Part print with two shaded views. Sizes in mm from the minimum x, y, z corner. A direction names the side the tool comes from. Round coordinates to 2 decimals unless told otherwise and drop trailing zeros. Order: outer loops, then holes, each group sorted by start corner. A loop starts at its lowest first (then second) coordinate and runs counter-clockwise, first axis right, second up. Notation, with made-up numbers: (28.5, 84.5) -> (36.5, 84.5) arc R15 cw to (36.5, 95.5) -> close; hole circle Ø2 at (50, 39.5). An arc over 180 degrees is marked (long way). Answer as a JSON object with one key per item and string values.
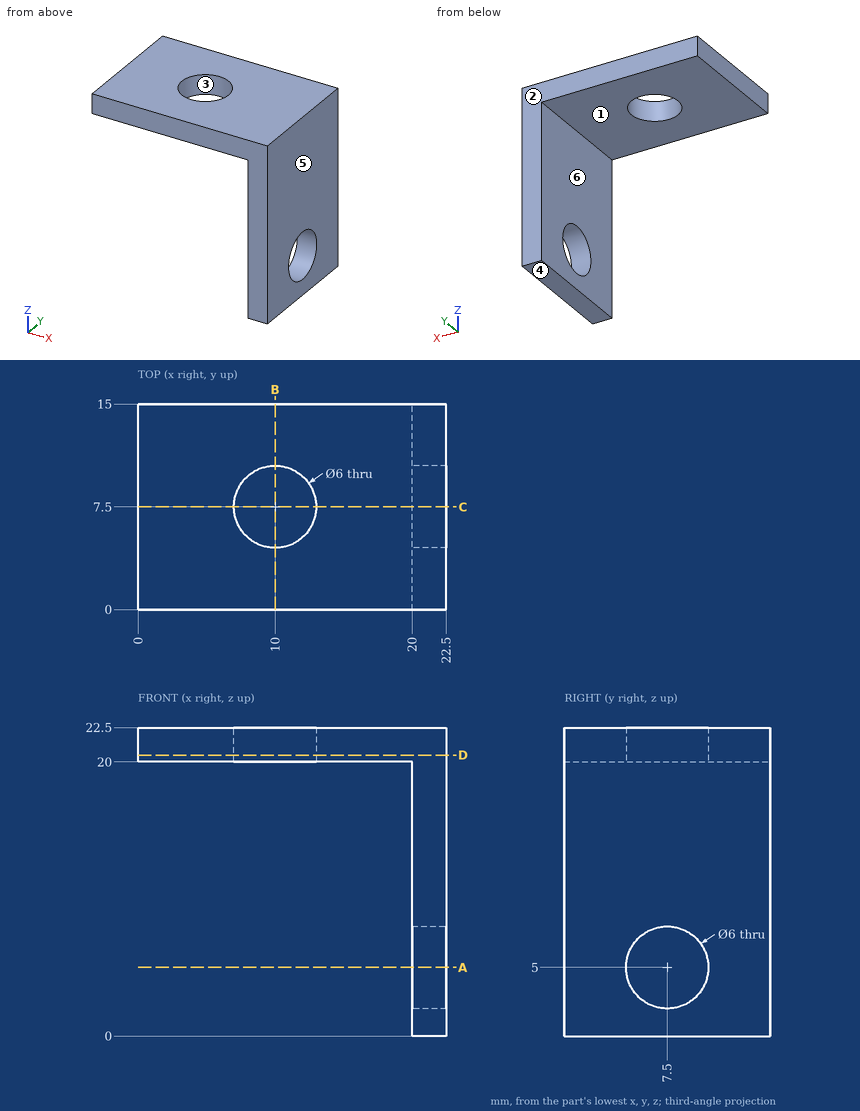
1) Cut at C-C, the plane y = 7.5. Give the cut face in (x, z).
Checked values:
{"outline": "(0, 20) -> (7, 20) -> (7, 22.5) -> (0, 22.5) -> close; (13, 20) -> (20, 20) -> (20, 8) -> (22.5, 8) -> (22.5, 22.5) -> (13, 22.5) -> close; (20, 0) -> (22.5, 0) -> (22.5, 2) -> (20, 2) -> close"}
2) Cut at D-D, the plane z = 20.5. Give the cut face in (x, y), plus the area to 3 significant figures.
Checked values:
{"outline": "(0, 0) -> (22.5, 0) -> (22.5, 15) -> (0, 15) -> close; hole circle Ø6 at (10, 7.5)", "area": "309 mm²"}
3) Probe L1, parallel to Y at x = 21.8, z = 5; L2, parallel to Z at x = 16.75, y = 3.25. List the from-to ranges inside material, lowest first. Write a range as from..to.
Checked values:
{"L1": "y = 0..4.5, 10.5..15", "L2": "z = 20..22.5"}
4) Cut at A-A, the plane z = 5. Give the cut face in (x, y), plus the area to 3 significant figures.
Checked values:
{"outline": "(20, 0) -> (22.5, 0) -> (22.5, 4.5) -> (20, 4.5) -> close; (20, 10.5) -> (22.5, 10.5) -> (22.5, 15) -> (20, 15) -> close", "area": "22.5 mm²"}
5) Which spindle directions (+Z, -Z, +X, -X, +Y, -Y) get a long thin tool onto all of the face, cutting with end or side? Do the marked faces 1 and 2. Say none if no direction does.
Checked values:
{"face 1": "-Z, -X, +Y, -Y", "face 2": "+Z, -Z, +X, -X, +Y"}
6) Cut at B-B, the plane x = 10. Give the cut face in (y, z).
Checked values:
{"outline": "(0, 20) -> (4.5, 20) -> (4.5, 22.5) -> (0, 22.5) -> close; (10.5, 20) -> (15, 20) -> (15, 22.5) -> (10.5, 22.5) -> close"}
7) Flat gauge pins, fed straight in: pin 1 Ø8 at (x, y) = (14, 3) entering from -Z; pin 2 Ø4.5 at (y, z) = (8, 7) entering from -X. Where does each tip first touch, or does it go through?
Checked values:
{"pin 1": "stops at z = 20", "pin 2": "stops at x = 20"}
8) Pull direction X, two halves, no side cores. Call the marked faces 3, 4, 5 and 6: pulls with the +X half, pulls with the -X half, needs draft (parallel to the pull), parting line crosses it, or undercut.
Checked values:
{"face 3": "undercut", "face 4": "needs draft", "face 5": "pulls with the +X half", "face 6": "pulls with the -X half"}
